Work out the finished part from the listing and answer in its coordinate system (mm). A direction names the side the tool comes from. Give positions to 0.01 mm unless a question says otherwise; leave off trailing zeros. Write each loop counter-clockwise with the first axis right and the second up, starting at its lowest first coordinate (ties: lowest second). Pieces come first, ordered by that corner, then holes.
1) Find section B-B (x = -12.5). Count the separate pieces of the cut face and the enclosed holes in it, plus the area to 3 significant figures.
2) A tool of negligible diameter and unlimited length cuts with its end or side. For faces 4 (the face through (0, -19, 16.66)), 5 (the face through (-24.797, 7.875, 20.431)), 6 (the face through (24.797, 15.138, -6.039)), from which of +Z, -Z, +X, -X, +Y, -Y can it reach the whole face along a straight path? Write none if from no direction.
3) Given pin 1 Ø5.5 at (x, y) = (11.5, -42) entering from +Z; pin 2 Ø4 at (x, z) = (-17.5, -29.5) entering from +Y; pin 3 Ø12 at (x, y) = (10, -45.5) entering from -Z, each flat-ended and moving along its own axis, determine where each tip first touches the part or whether it passes through.
4) Straight lines are drawn through the part: probe 1 along X at (y, z) = (-43, 2); probe 2 along Z at (x, y) = (16.5, -26); probe 3 along Y at (x, z) = (12, 13). For each, find the intervals that lie inside material, in ascending order.
5) Determine the mould class of faces 1 (the face through (0, -23, -4)), 2 (the face through (24.8, 8.31, 35.98)), 3 (the face through (0, -37.29, 4)) for opening direction Y: pulls with the +Y half, pulls with the -Y half, needs draft (parallel to the pull), parting line crosses it, or undercut.
6) Find section A-A (y = -15). Determine the outline of the cut face in (x, z), plus the area to 3 significant figures.
7) Find section D-D (z = -64.5). Determine the outline of the cut face in (x, y).
```python
from build123d import *

# Parameters (mm, degrees)
SKETCH1_W               = 8
SKETCH1_H               = 11.83
BOSS_EXTRUDE1_DEPTH     = 25
CUT_EXTRUDE1_DEPTH      = 119.472964421
CUT_EXTRUDE1_DEPTH_BACK = 119.472964421
FILLET1_R               = 2
FILLET2_R               = 0.5
CHAMFER1_SIZE           = 0.4
FILLET3_R               = 0.2
CHAMFER2_SIZE           = 0.4


with BuildPart() as part:
    # Sketch1 → Boss-Extrude1 (new body)
    with BuildSketch(Plane.YZ):
        Polygon((-41.29, -4), (4, -4), (4, 0.618802154), (4, 5.205186779), (4, 20.66), (-41.29, 20.66), (-41.29, 8.83), (-37.29, 8.83), (-37.29, 16.66), (0, 16.66), (0, 0), (-37.29, 0), (-37.29, 7.83), (-41.29, 7.83), align=None)
        Polygon((4, 0.618802154), (4, -4), (30.836144658, -19.493855342), (50.861332538, -94.228873943), (54.725035843, -93.193597763), (15.902179078, 51.69527618), (12.038475773, 50.66), (4, 20.66), (4, 5.205186779), (14.109028134, 42.93259339), (29.372043043, -14.029753727), align=None)
        with Locations((-45.29, 14.745)):
            Rectangle(SKETCH1_W, SKETCH1_H)
        with Locations((-45.29, 1.915)):
            Rectangle(SKETCH1_W, SKETCH1_H)
    extrude(amount=BOSS_EXTRUDE1_DEPTH)

    # Sketch2 → Cut-Extrude1 (cut, two sides: drawn at the far end of the back side and taken through both)
    with BuildSketch(Plane.XY.offset(7.83).offset(-CUT_EXTRUDE1_DEPTH_BACK)):
        with BuildLine():
            ThreePointArc((9.3, -43.29), (12.5, -46.49), (15.7, -43.29))
            Line((15.7, -43.29), (9.3, -43.29))
        make_face()
        with BuildLine():
            Line((9.3, -43.29), (15.7, -43.29))
            ThreePointArc((15.7, -43.29), (12.5, -40.09), (9.3, -43.29))
        make_face()
    extrude(amount=CUT_EXTRUDE1_DEPTH + CUT_EXTRUDE1_DEPTH_BACK, mode=Mode.SUBTRACT)

    # Fillet1
    fillet1_edges = [part.edges().sort_by_distance(p)[0] for p in [
        (12.5, 4, -4),
        (12.5, 30.836144658, -19.493855342),
        (12.5, 50.861332538, -94.228873943),
        (12.5, 54.725035843, -93.193597763),
        (12.5, 15.902179078, 51.69527618),
        (12.5, 12.038475773, 50.66),
        (12.5, 14.109028134, 42.93259339),
        (12.5, 29.372043043, -14.029753727),
        (12.5, 4, 0.618802154),
        (12.5, 4, 5.205186779),
        (12.5, 4, 20.66),
    ]]
    fillet(fillet1_edges, radius=FILLET1_R - 0.0001)  # a hair under: the kernel refuses the full size

    # Fillet2
    fillet2_edges = [part.edges().sort_by_distance(p)[0] for p in [
        (12.5, -37.29, 8.83),
        (12.5, -49.29, 8.83),
        (12.5, -49.29, 20.66),
        (12.5, -49.29, -4),
        (12.5, -49.29, 7.83),
        (12.5, -37.29, 7.83),
    ]]
    fillet(fillet2_edges, radius=FILLET2_R)

    # Chamfer1
    chamfer1_edges = [part.edges().sort_by_distance(p)[0] for p in [
        (15.7, -43.29, 7.83),
        (15.7, -43.29, -4),
        (15.7, -43.29, 20.66),
        (15.7, -43.29, 8.83),
    ]]
    chamfer(chamfer1_edges, length=CHAMFER1_SIZE)

    # Mirror1: part across plane


with BuildPart() as part_1:
    add(part.part)
    add(part.part.mirror(Plane(origin=(0, 0, 0), x_dir=(0, 0, 1), z_dir=(1, 0, 0))))

    # Fillet3
    fillet3_edges = [part_1.edges().sort_by_distance(p)[0] for p in [
        (0, -37.29, 0),
        (0, 0, 0),
        (0, 0, 16.66),
        (0, -37.29, 16.66),
    ]]
    fillet(fillet3_edges, radius=FILLET3_R)

    # Chamfer2
    chamfer2_edges = [part_1.edges().sort_by_distance(p)[0] for p in [
        (25, 54.00763278, -92.779404911),
        (25, 51.27552539, -93.51147088),
        (25, 3.981740618, -4.06814494),
        (25, 30.70541894, -19.594164714),
        (25, 14.109028134, 37.20547315),
        (25, 27.408123551, -11.470324016),
        (25, 4.267935795, 0.773494957),
        (25, 4.017109422, 5.202934281),
        (25, 3.682884739, 21.073272655),
        (25, -43.29, 7.83),
        (25, -49.29, 14.745),
        (25, -43.29, 8.83),
        (25, -37.29, 12.895),
        (25, -49.29, 1.915),
        (25, -49.143553391, 20.513553391),
        (25, -49.143553391, -3.853553391),
        (25, -49.143553391, 8.976446609),
        (25, -49.143553391, 7.683553391),
        (25, -37.436446609, 8.976446609),
        (25, -37.436446609, 7.683553391),
        (-25, -43.29, 7.83),
        (-25, -49.29, 1.915),
        (-25, 17.291410002, -11.673799143),
        (-25, 40.697133492, -56.295566685),
        (-25, 35.313607461, -20.749160791),
        (-25, 13.562099547, 51.06825376),
        (-25, 8.068405021, 35.843494244),
        (-25, -23.162288622, 20.66),
        (-25, -37.29, 12.895),
        (-25, 15.095330785, -5.787090062),
        (-25, 4, 3.357669953),
        (-25, 8.122709007, 20.591346258),
        (-25, 22.081599912, 13.178550448),
        (-25, -43.29, 8.83),
        (-25, -49.29, 14.745),
        (-25, -22.662935795, -4),
        (-25, 3.981740618, -4.06814494),
        (-25, 30.70541894, -19.594164714),
        (-25, 54.00763278, -92.779404911),
        (-25, 51.27552539, -93.51147088),
        (-25, 15.487986226, 50.977873117),
        (-25, 12.257244433, 50.441231339),
        (-25, 14.109028134, 37.20547315),
        (-25, 27.408123551, -11.470324016),
        (-25, 4.267935795, 0.773494957),
        (-25, 4.017109422, 5.202934281),
        (-25, 3.682884739, 21.073272655),
        (-25, -37.436446609, 7.683553391),
        (-25, -37.436446609, 8.976446609),
        (-25, -49.143553391, 7.683553391),
        (-25, -49.143553391, 8.976446609),
        (-25, -49.143553391, -3.853553391),
        (-25, -49.143553391, 20.513553391),
        (-25, -18.645, 0),
        (25, -18.645, 0),
        (-25, 0, 8.33),
        (25, 0, 8.33),
        (-25, -37.29, 3.765),
        (25, -37.29, 3.765),
        (-25, -18.645, 16.66),
        (25, -18.645, 16.66),
        (-25, -0.058578644, 0.058578644),
        (25, -0.058578644, 0.058578644),
        (-25, -37.231421356, 0.058578644),
        (25, -37.231421356, 0.058578644),
        (-25, -37.231421356, 16.601421356),
        (25, -37.231421356, 16.601421356),
        (-25, -0.058578644, 16.601421356),
        (25, -0.058578644, 16.601421356),
        (25, 17.291410002, -11.673799143),
        (25, -22.662935795, -4),
        (25, 40.697133492, -56.295566685),
        (25, 15.095330785, -5.787090062),
        (25, 4, 3.357669953),
        (25, 8.122709007, 20.591346258),
        (25, 22.081599912, 13.178550448),
        (25, 35.313607461, -20.749160791),
        (25, 13.562099547, 51.06825376),
        (25, 8.068405021, 35.843494244),
        (25, -23.162288622, 20.66),
        (25, 12.257244433, 50.441231339),
        (25, 15.487986226, 50.977873117),
    ]]
    chamfer(chamfer2_edges, length=CHAMFER2_SIZE)


solid = part_1.part
```
Results:
1. separate pieces: 3
1. enclosed holes: 1
1. area: 1,400 mm2
2. face 4: +X, -X
2. face 5: -X
2. face 6: +X
3. pin 1: stops at z = 20.66
3. pin 2: stops at y = 38.19
3. pin 3: stops at z = -4
4. probe 1: x = -25 to -15.69, -9.31 to 9.31, 15.69 to 25
4. probe 2: z = -4 to 0, 16.66 to 20.66
4. probe 3: y = -49.29 to -46.45, -40.13 to -37.29, 0 to 6.09, 22.13 to 26.27
5. face 1: needs draft
5. face 2: pulls with the -Y half
5. face 3: undercut
6. outline: (-25, -3.6) - (-24.6, -4) - (24.6, -4) - (25, -3.6) - (25, -0.4) - (24.6, 0) - (-24.6, 0) - (-25, -0.4) - close; (-25, 17.06) - (-24.6, 16.66) - (24.6, 16.66) - (25, 17.06) - (25, 20.26) - (24.6, 20.66) - (-24.6, 20.66) - (-25, 20.26) - close
6. area: 399 mm2
7. outline: (-25, 43.31) - (-24.6, 42.9) - (24.6, 42.9) - (25, 43.31) - (25, 46.62) - (24.6, 47.04) - (-24.6, 47.04) - (-25, 46.62) - close
